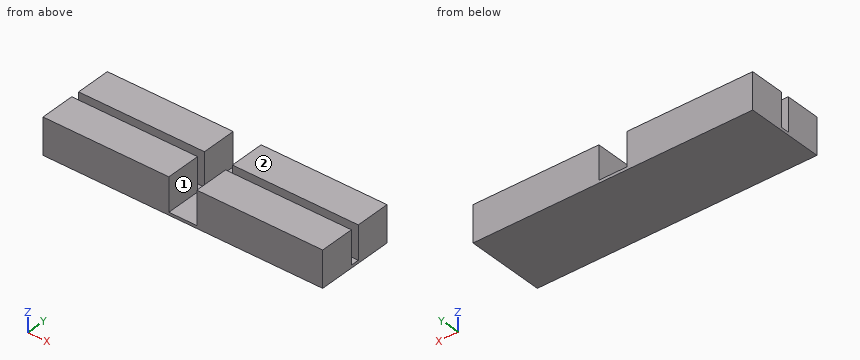
```python
from build123d import *

# Parameters (mm, degrees)
SKETCH_1_W          = 20
SKETCH_1_H          = 5.6
EXTRUDE_1_DEPTH     = 2.6
SKETCH_2_W          = 2.4
SKETCH_2_H          = 0.6
CUT_EXTRUDE_1_DEPTH = 21
SKETCH_3_W          = 2
SKETCH_3_H          = 2.4
CUT_EXTRUDE_2_DEPTH = 6.6


with BuildPart() as part:
    # 草图1 → 凸台-拉伸1 (new body)
    with BuildSketch(Plane.XY):
        Rectangle(SKETCH_1_W, SKETCH_1_H)
    extrude(amount=EXTRUDE_1_DEPTH)

    # 草图2 → 切除-拉伸1 (cut, through all)
    with BuildSketch(Plane(origin=(10, 0, 0), x_dir=(0, 0, -1), z_dir=(1, 0, 0))):
        with Locations((-1.4, 0)):
            Rectangle(SKETCH_2_W, SKETCH_2_H)
    extrude(amount=-CUT_EXTRUDE_1_DEPTH, mode=Mode.SUBTRACT)

    # 草图3 → 切除-拉伸2 (cut, through all)
    with BuildSketch(Plane.XZ.offset(2.8)):
        with Locations((0, 1.4)):
            Rectangle(SKETCH_3_W, SKETCH_3_H)
    extrude(amount=-CUT_EXTRUDE_2_DEPTH, mode=Mode.SUBTRACT)


solid = part.part
```
Verification items for the finished model (mm, model axes). Face numbers are marked on the shaded views. A direction names the side the tool comes from. Round coordinates to 2 decimals unless told otherwise and drop trailing zeros. Loops run counter-clockwise (first coordinate to the right, second up) from the corner with the lowest first, then second, coordinate; pieces in that order, holes last. Notation, with made-up numbers: (76.25, 89.25) -> (93.25, 89.25) arc R13 cw to (93.25, 93.25) -> close; hole circle Ø6 at (73.5, 75). An arc over 180 degrees is marked (long way). Answer as a JSON object with one key per item and string values.
Q1. Section check C-C (y = -2.3). Record the boundary of the cut face in (x, z), then the cut area to 3 significant figures.
Data:
{"outline": "(-10, 0) -> (10, 0) -> (10, 2.6) -> (1, 2.6) -> (1, 0.2) -> (-1, 0.2) -> (-1, 2.6) -> (-10, 2.6) -> close", "area": "47.2 mm2"}
Q2. Scan lines: line 1 (Y direction, x = 8.25, z = 0.3); line 2 (X direction, y = 1.55, z = 1.1); line 3 (Z direction, x = -7.25, y = -0.1). Record each from-to range of solid material in increasing order. Write a range as from..to.
Data:
{"line 1": "y = -2.8..-0.3, 0.3..2.8", "line 2": "x = -10..-1, 1..10", "line 3": "z = 0..0.2"}
Q3. Section check A-A (z = 2.15). Record the boundary of the cut face in (x, y).
Data:
{"outline": "(-10, -2.8) -> (-1, -2.8) -> (-1, -0.3) -> (-10, -0.3) -> close; (-10, 0.3) -> (-1, 0.3) -> (-1, 2.8) -> (-10, 2.8) -> close; (1, -2.8) -> (10, -2.8) -> (10, -0.3) -> (1, -0.3) -> close; (1, 0.3) -> (10, 0.3) -> (10, 2.8) -> (1, 2.8) -> close"}
Q4. Section check B-B (x = -2.25). Record the boundary of the cut face in (y, z), then the cut area to 3 significant figures.
Data:
{"outline": "(-2.8, 0) -> (2.8, 0) -> (2.8, 2.6) -> (0.3, 2.6) -> (0.3, 0.2) -> (-0.3, 0.2) -> (-0.3, 2.6) -> (-2.8, 2.6) -> close", "area": "13.1 mm2"}
Q5. Access from +Z, -Z, +X, -X, +Y, -Y to the whole of each face (thin tool, end or side, straight path). Record for the marked faces 1 and 2.
Data:
{"face 1": "+Z, +Y, -Y", "face 2": "+Z, +X, -X, +Y, -Y"}
